Here's how the part is built. I have some questions about the finished solid (model axes, mm). Face numbers are marked on the shaded views. A direction names the side the tool comes from. Coordinates: 2 decimals unless noted, no trailing zeros. Write each loop counter-clockwise with the first axis right and the second up, starting at its lowest first coordinate (ties: lowest second). Pieces come first, ordered by that corner, then holes.
Item 1: We'd pull the mould along Y, two halves only. Please class the marked faces 1, 2 and 3: +Y half, -Y half, draft (parallel to the pull), parting line (faces both ways), or undercut.
Item 2: If we section it at C-C (x = 51.5): Please give me the cut outline in (y, z).
Item 3: If we section it at D-D (y = 37.5): Please give me the cut outline in (x, z) (3 decimals), then the cut area to 3 significant figures.
Item 4: For the marked faces 4, 5 and 6, which set-ups out of +Z, -Z, +X, -X, +Y, -Y let a thin tool reach every point of the face, with its end or its side?
Item 5: I'm going to push a flat-ended pin straight in: pin 1 Ø4 at (x, z) = (12.5, 12.5) entering from +Y. Where does the tip first touch, or does it pass through?
Item 6: If I drill on line 1 (Z direction, x = 50.5, y = 21); line 2 (X direction, y = 17, z = 2.75); line 3 (X direction, y = 38.5, z = 15.75), over which ranges is the centre line in solid material (lowest first)?
Item 7: If we section it at B-B (z = 10.25): Please give me the cut outline in (x, y), then the cut area to 3 significant figures.
Item 8: If we section it at A-A (y = 12): Please give me the cut outline in (x, z) (3 decimals), then the cut area to 3 significant figures.
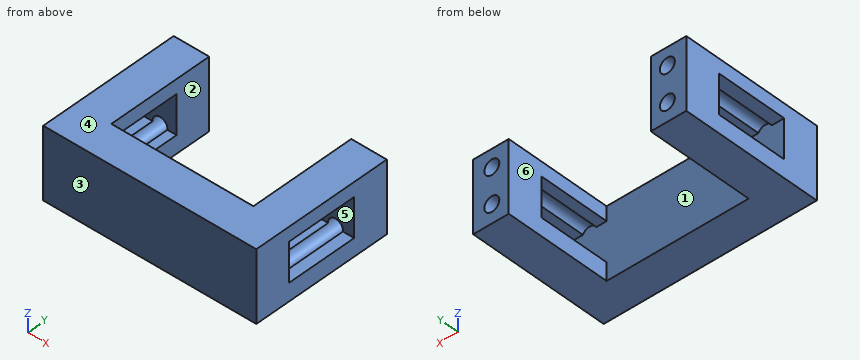
from build123d import *

# Parameters (mm, degrees)
SKIZZE1_W                       = 60
SKIZZE1_H                       = 40
AUFSATZ_LINEAR_AUSTRAGEN1_DEPTH = 20
SKIZZE2_W                       = 40
SKIZZE2_H                       = 20
SCHNITT_LINEAR_AUSTRAGEN1_DEPTH = 30
SKIZZE3_W                       = 11
SKIZZE3_H                       = 20
SCHNITT_LINEAR_AUSTRAGEN2_DEPTH = 61
SKIZZE4_R                       = 2.1
SCHNITT_LINEAR_AUSTRAGEN3_DEPTH = 30


with BuildPart() as part:
    # Skizze1 → Aufsatz-Linear austragen1 (new body)
    with BuildSketch(Plane.XY):
        with Locations((30, 20)):
            Rectangle(SKIZZE1_W, SKIZZE1_H)
    extrude(amount=AUFSATZ_LINEAR_AUSTRAGEN1_DEPTH)

    # Skizze2 → Schnitt-Linear austragen1 (cut)
    with BuildSketch(Plane(origin=(0, 40, 0), x_dir=(1, 0, 0), z_dir=(0, 1, 0))):
        with Locations((30, -10)):
            Rectangle(SKIZZE2_W, SKIZZE2_H)
    extrude(amount=-SCHNITT_LINEAR_AUSTRAGEN1_DEPTH, mode=Mode.SUBTRACT)

    # Skizze3 → Schnitt-Linear austragen2 (cut, through all)
    with BuildSketch(Plane(origin=(60, 0, 0), x_dir=(0, 0, -1), z_dir=(1, 0, 0))):
        with Locations((-10.5, 20)):
            Rectangle(SKIZZE3_W, SKIZZE3_H)
    extrude(amount=-SCHNITT_LINEAR_AUSTRAGEN2_DEPTH, mode=Mode.SUBTRACT)

    # Skizze4 → Schnitt-Linear austragen3 (cut)
    with BuildSketch(Plane(origin=(0, 40, 0), x_dir=(1, 0, 0), z_dir=(0, 1, 0))):
        with Locations((5.338854382, -5.225)):
            Circle(SKIZZE4_R)
        with Locations((5.338854382, -15.075)):
            Circle(SKIZZE4_R)
        with Locations((54.761145618, -15.075)):
            Circle(SKIZZE4_R)
        with Locations((54.761145618, -5.225)):
            Circle(SKIZZE4_R)
    extrude(amount=-SCHNITT_LINEAR_AUSTRAGEN3_DEPTH, mode=Mode.SUBTRACT)


solid = part.part
Answer list:
1. face 1: undercut
1. face 2: draft
1. face 3: -Y half
2. outline: (0, 0) - (40, 0) - (40, 20) - (0, 20) - close; hole (10, 5) - (30, 5) - (30, 16) - (10, 16) - close
3. outline: (0, 0) - (10, 0) - (10, 20) - (0, 20) - close; (50, 0) - (60, 0) - (60, 20) - (50, 20) - close; hole circle Ø4.2 at (5.339, 5.225); hole circle Ø4.2 at (5.339, 15.075); hole circle Ø4.2 at (54.761, 5.225); hole circle Ø4.2 at (54.761, 15.075)
3. area: 345 mm2
4. face 4: +Z, +X, -X, +Y, -Y
4. face 5: +X, -X
4. face 6: +Z, -Z, +Y
5. pin 1: stops at y = 10
6. line 1: z = 0 to 5, 16 to 20
6. line 2: x = 0 to 10, 50 to 60
6. line 3: x = 0 to 3.35, 7.33 to 10, 50 to 52.77, 56.75 to 60
7. outline: (0, 0) - (60, 0) - (60, 10) - (0, 10) - close; (0, 30) - (10, 30) - (10, 40) - (0, 40) - close; (50, 30) - (60, 30) - (60, 40) - (50, 40) - close
7. area: 800 mm2
8. outline: (0, 0) - (10, 0) - (10, 5) - (7.427, 5) arc R2.1 cw to (3.251, 5) - (0, 5) - close; (0, 16) - (3.454, 16) arc R2.1 cw to (7.224, 16) - (10, 16) - (10, 20) - (0, 20) - close; (50, 0) - (60, 0) - (60, 5) - (56.849, 5) arc R2.1 cw to (52.673, 5) - (50, 5) - close; (50, 16) - (52.876, 16) arc R2.1 cw to (56.646, 16) - (60, 16) - (60, 20) - (50, 20) - close
8. area: 162 mm2
